from build123d import *

# Parameters (mm, degrees)
F0_W     = 2
F0_H     = 5
F1_DEPTH = 66
F2_R     = 1
F3_R     = 1


with BuildPart() as f1:
    # F0 (on Right) → F1 (new body)
    with BuildSketch(Plane.YZ):
        Polygon((-33.5, 0), (0, 0), (33.5, 0), (35.5, 0), (40, 0), (42, 0), (0, 90), (-42, 0), (-42, -5), (-40, -5), (-40, 0), (-35.5, 0), (-35.5, -5), (-33.5, -5), align=None)
        Polygon((38.859607, 2), (0, 2), (-38.859607, 2), (0, 85.270587), align=None, mode=Mode.SUBTRACT)
        with Locations((34.5, -2.5)):
            Rectangle(F0_W, F0_H)
        with Locations((41, -2.5)):
            Rectangle(F0_W, F0_H)
    extrude(amount=F1_DEPTH)

    # F2
    f2_edges = [f1.edges().sort_by_distance(p)[0] for p in [
        (33, 0, 90),
    ]]
    fillet(f2_edges, radius=F2_R)

    # F3
    f3_edges = [f1.edges().sort_by_distance(p)[0] for p in [
        (33, 0, 85.270587),
        (33, 38.859607, 2),
        (33, -38.859607, 2),
    ]]
    fillet(f3_edges, radius=F3_R)


solid = f1.part
Verification items for the finished model (mm, model axes). A direction names the side the tool comes from. Coordinates: 2 decimals unless noted, no trailing zeros. Write each loop counter-clockwise with the first axis right and the second up, starting at its lowest first coordinate (ties: lowest second). Pieces come first, ordered by that corner, then holes. Notation, with made-up numbers: (31, -13) - (53, -13) arc R25 cw to (53, 1) - close; hole circle Ø8 at (44.5, 28.5). An arc over 180 degrees is marked (long way). Answer as a JSON object with one key per item and string values.
(1) Thickness scan on line 1 along Z through (x, y) = (43, 34); line 2 along Z through (x, y) = (43, -21); line 3 along Y through (x, z) = (46, 33). Record the ranges inside material, lowest first.
Report:
{"line 1": "-5 to 2, 12.41 to 17.14", "line 2": "0 to 2, 40.27 to 45", "line 3": "-26.6 to -24.39, 24.39 to 26.6"}
(2) Gauge pin test, flat ends, axial feed: pin 1 Ø1.3 at (x, y) = (31.5, 38) entering from -Z; pin 2 Ø2 at (x, z) = (50, 47.5) entering from +Y; pin 3 Ø3 at (x, y) = (36.5, 28.5) entering from +Z. Record the tip position at first contact, or that the pin passes through.
Report:
{"pin 1": "z = 0", "pin 2": "y = 20.3", "pin 3": "z = 32.14"}
(3) Cross-section at C-C on z = 27. Record the cut outline in (x, y), plus the area to 3 significant figures.
Report:
{"outline": "(0, -29.4) - (66, -29.4) - (66, -27.19) - (0, -27.19) - close; (0, 27.19) - (66, 27.19) - (66, 29.4) - (0, 29.4) - close", "area": "291 mm^2"}
(4) Mould release check, pull along Y, two halves, no side actions. Record for faces 4 (the flat face through (33, 42, -3)), 5 (the flat face through (33, -21, 45)), 6 (the flat face through (33, -40, -3)): pulls with the +Y half, pulls with the -Y half, needs draft (parallel to the pull), parting line crosses it, or undercut.
Report:
{"face 4": "pulls with the +Y half", "face 5": "pulls with the -Y half", "face 6": "undercut"}
(5) Cross-section at A-A on x = 50. Record the cut outline in (y, z), plus the area to 3 significant figures.
Report:
{"outline": "(-42, -5) - (-40, -5) - (-40, 0) - (-35.5, 0) - (-35.5, -5) - (-33.5, -5) - (-33.5, 0) - (33.5, 0) - (33.5, -5) - (35.5, -5) - (35.5, 0) - (40, 0) - (40, -5) - (42, -5) - (42, 0) - (0.91, 88.06) arc R1 ccw to (-0.91, 88.06) - (-42, 0) - close; hole (-38.2, 3.42) arc R1 ccw to (-37.29, 2) - (37.29, 2) arc R1 ccw to (38.2, 3.42) - (0.91, 83.33) arc R1 ccw to (-0.91, 83.33) - close", "area": "585 mm^2"}
(6) Cross-section at B-B on y = 28.5. Record the cut outline in (x, z), plus the area to 3 significant figures.
Report:
{"outline": "(0, 0) - (66, 0) - (66, 2) - (0, 2) - close; (0, 24.2) - (66, 24.2) - (66, 28.93) - (0, 28.93) - close", "area": "444 mm^2"}
(7) Tool access check on faces 1 (the flat face through (66, -22, 39)), 2 (the flat face through (32.538, 19.29, 43.935)), 3 (the flat face through (33, 38, 0)). Record the directions out of +Z, -Z, +X, -X, +Y, -Y that give a thin tool (end or side, any length) a straight path to the whole face; none if there is none.
Report:
{"face 1": "+Z, -Z, +X, +Y, -Y", "face 2": "+X, -X", "face 3": "-Z, +X, -X"}
